```python
from build123d import *

# Parameters (mm, degrees)
SKETCH1_W           = 183
SKETCH1_H           = 77
BOSS_EXTRUDE1_DEPTH = 57
FILLET1_R           = 4
SKETCH2_R           = 19.259927961
CUT_EXTRUDE1_DEPTH  = 42


with BuildPart() as part:
    # Sketch1 → Boss-Extrude1 (new body)
    with BuildSketch(Plane(origin=(0, 0, 0), x_dir=(1, 0, 0), z_dir=(0, 1, 0))):
        with Locations((-105.718045113, 24.105263158)):
            Rectangle(SKETCH1_W, SKETCH1_H)
    extrude(amount=BOSS_EXTRUDE1_DEPTH)

    # Fillet1
    fillet1_edges = [part.edges().sort_by_distance(p)[0] for p in [
        (-14.218045113, 57, -24.105263158),
        (-105.718045113, 57, -62.605263158),
        (-197.218045113, 57, -24.105263158),
        (-105.718045113, 0, -62.605263158),
        (-14.218045113, 0, -24.105263158),
        (-105.718045113, 0, 14.394736842),
        (-197.218045113, 0, -24.105263158),
        (-105.718045113, 57, 14.394736842),
        (-197.218045113, 28.5, -62.605263158),
        (-14.218045113, 28.5, -62.605263158),
        (-14.218045113, 28.5, 14.394736842),
        (-197.218045113, 28.5, 14.394736842),
    ]]
    fillet(fillet1_edges, radius=FILLET1_R)

    # Sketch2 → Cut-Extrude1 (cut, symmetric)
    with BuildSketch(Plane(origin=(-105.718045113, 0, 0), x_dir=(0, 0, -1), z_dir=(1, 0, 0))):
        with Locations(Location((25.391658687, 29.2539915, 0), (0, 0, 180))):
            Circle(SKETCH2_R)
    extrude(amount=CUT_EXTRUDE1_DEPTH, both=True, mode=Mode.SUBTRACT)


solid = part.part
```
Part model, mm, in its own coordinate system. A direction names the side the tool comes from. Round coordinates to 2 decimals unless told otherwise and drop trailing zeros. Order: outer loops, then holes, each group sorted by start corner. A loop starts at its lowest first (then second) coordinate and runs counter-clockwise, first axis right, second up. Notation, with made-up numbers: M -1,87.25 L 41,87.25 A26 ccw 41,108.25 Z; hole C 55,68 d9. An arc over 180 degrees is marked long. Answer in a Markdown table with one row per item. Add a question column.
Q1. Cut at A-A on y = 45. Give the cut face in (x, z).
Q2. Cut at B-B on z = -15.5. Give the cut face in (x, y).
Q3. Cut at C-C on x = -73.5. Give the cut face in (y, z).
Q4. Mould opens along Z. For faces 3 (the face through (-147.718, 29, -26)), 4 (the face through (-104.49, 1.2, -61.46)), 5 (the face through (-15.36, 55.8, -24.59)) say: +Z half, -Z half, draft (parallel to the pull), parting line (faces both ways), or undercut.
Q5. 3-axis set-ups, long thin cutter, end or side, ignore diameter. For faces 1 (the face through (-15.421, 28.843, 13.254)), 2 (the face through (-63.718, 29, -26)): which of +Z, -Z, +X, -X, +Y, -Y reach the whole face in a straight line?
Q6. Wall check: L1, parallel to X at y = 26, z = -40.5; L2, parallel to Z at x = -72.5, y = 46; L3, parallel to Z at x = -122, y = 13.5. Give the ranges that are in metal, low to high. Write a range as from..to.
Established:
| question | item | result |
|---|---|---|
| 1 | outline | M -197.22,-58.61 A4 ccw -193.22,-62.61 L -18.22,-62.61 A4 ccw -14.22,-58.61 L -14.22,10.39 A4 ccw -18.22,14.39 L -193.22,14.39 A4 ccw -197.22,10.39 Z; hole M -147.72,-36.48 L -63.72,-36.48 L -63.72,-14.3 L -147.72,-14.3 Z |
| 2 | outline | M -197.22,4 A4 ccw -193.22,0 L -18.22,0 A4 ccw -14.22,4 L -14.22,53 A4 ccw -18.22,57 L -193.22,57 A4 ccw -197.22,53 Z; hole M -147.72,12.73 L -63.72,12.73 L -63.72,45.78 L -147.72,45.78 Z |
| 3 | outline | M 0,-58.61 A4 ccw 4,-62.61 L 53,-62.61 A4 ccw 57,-58.61 L 57,10.39 A4 ccw 53,14.39 L 4,14.39 A4 ccw 0,10.39 Z; hole C 29.25,-25.39 d38.52 |
| 4 | face 3 | undercut |
| 4 | face 4 | -Z half |
| 4 | face 5 | draft |
| 5 | face 1 | +Z, +X, +Y, -Y |
| 5 | face 2 | none |
| 6 | L1 | x = -197.22..-147.72, -63.72..-14.22 |
| 6 | L2 | z = -62.61..-34.91, -15.88..14.39 |
| 6 | L3 | z = -62.61..-36.47, -14.31..14.39 |
